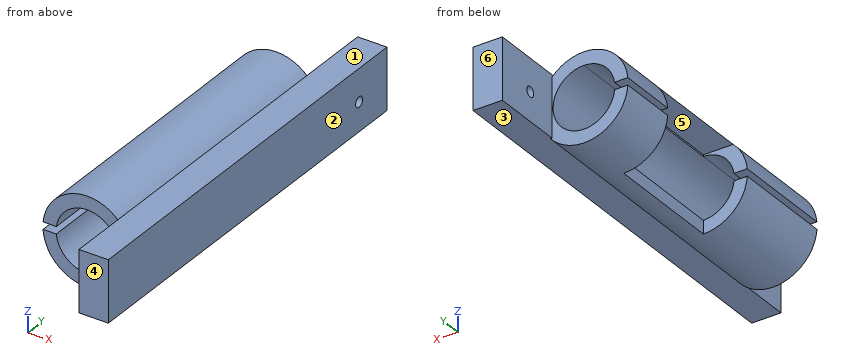
```python
from build123d import *

# Parameters (mm, degrees)
SKETCH_1_R           = 15
EXTRUDE_1_DEPTH      = 95
SKETCH_2_R           = 10.5
CUT_EXTRUDE_1_DEPTH  = 95
EXTRUDE_2_DEPTH      = 20
EXTRUDE_2_DEPTH_BACK = 120
SKETCH_3_W           = 10
SKETCH_3_H           = 20.861334049
SKETCH_7_W           = 15
SKETCH_7_H           = 40
CUT_EXTRUDE_3_DEPTH  = 125.54811794
SKETCH_8_W           = 8.046060948
SKETCH_8_H           = 2.469161561
CUT_EXTRUDE_4_DEPTH  = 118.826105551
SKETCH_10_R          = 1.75
CUT_EXTRUDE_5_DEPTH  = 124.649640842


with BuildPart() as part:
    # 草图1 → 凸台-拉伸1 (new body)
    with BuildSketch(Plane(origin=(0, 0, 0), x_dir=(1, 0, 0), z_dir=(0, 1, 0))):
        with Locations(Location((0, 0, 0), (0, 0, 270))):
            Circle(SKETCH_1_R)
    extrude(amount=EXTRUDE_1_DEPTH)

    # 草图2 → 切除-拉伸1 (cut)
    with BuildSketch(Plane(origin=(0, 95, 0), x_dir=(1, 0, 0), z_dir=(0, 1, 0))):
        with Locations(Location((0, 0, 0), (0, 0, 270))):
            Circle(SKETCH_2_R)
    extrude(amount=-CUT_EXTRUDE_1_DEPTH, mode=Mode.SUBTRACT)

    # 草图3 → 凸台-拉伸2 (add, two sides: drawn at the far end of the back side and taken through both)
    with BuildSketch(Plane(origin=(0, 0, 0), x_dir=(-1, 0, 0), z_dir=(0, -1, 0)).offset(-EXTRUDE_2_DEPTH_BACK)):
        with Locations((-15.808439379, -0.631614786)):
            Rectangle(SKETCH_3_W, SKETCH_3_H)
    extrude(amount=EXTRUDE_2_DEPTH + EXTRUDE_2_DEPTH_BACK)

    # 草图7 → 切除-拉伸3 (cut, through all)
    with BuildSketch(Plane.XY.offset(11.06228181)):
        with Locations((-7.5, 55)):
            Rectangle(SKETCH_7_W, SKETCH_7_H)
    extrude(amount=-CUT_EXTRUDE_3_DEPTH, mode=Mode.SUBTRACT)

    # 草图8 → 切除-拉伸4 (cut, through all)
    with BuildSketch(Plane(origin=(0, 95, 0), x_dir=(1, 0, 0), z_dir=(0, 1, 0))):
        with Locations((-13.909114393, -0.200189033)):
            Rectangle(SKETCH_8_W, SKETCH_8_H)
    extrude(amount=-CUT_EXTRUDE_4_DEPTH, mode=Mode.SUBTRACT)

    # 草图10 → 切除-拉伸5 (cut, through all)
    with BuildSketch(Plane.ZY.offset(-10.808439379)):
        with Locations((0, 106)):
            Circle(SKETCH_10_R)
    extrude(amount=-CUT_EXTRUDE_5_DEPTH, mode=Mode.SUBTRACT)


solid = part.part
```
CAD build for the part. Positions are in the model's coordinates, mm. Face numbers are marked on the shaded views. A direction names the side the tool comes from. Round coordinates to 2 decimals unless told otherwise and drop trailing zeros. Loops run counter-clockwise (first coordinate to the right, second up) from the corner with the lowest first, then second, coordinate; pieces in that order, holes last. Notation, with made-up numbers: (-24, 26.5) - (-20, 26.5) arc R25 ccw to (-20, 61.5) - close; hole circle Ø2 at (-19, 62). An arc over 180 degrees is marked (long way). Return JSON: item names as keys, results as strings. Group by question number.
Q1. Flat gauge pins, fed straight in: pin 1 Ø2 at (x, z) = (9, 12) entering from +Y; pin 2 Ø3 at (x, y) = (16, 20) entering from -Z; pin 3 Ø3.5 at (x, y) = (-12, 85) entering from +Z. Where does each tip first touch, or does it go through?
Q2. Band-saw the part on D-D on x = 15. Give the cut face in (y, z), plus the area to 3 significant figures.
Q3. Drill centre lines: line 1 along Z through (x, y) = (-0.5, 10); line 2 along X through (y, z) = (107.5, 5.75); line 3 along Z through (x, y) = (1.5, 22). Where is each one in solid material? Low to high. Write a range as [from, to].
Q4. Tool access for the marked faces 1 and 2: list every direction of +Z, -Z, +X, -X, +Y, -Y with a clear straight run to the whole face (end or side of a thin tool).
Q5. Band-saw the part on C-C on z = 5.25. Give the cut face in (x, y).
Q6. Band-saw the part on A-A on x = -12. Give the cut face in (y, z), plus the area to 3 significant figures.
Q7. Two-plate mould, pull along Y, no slides. Class the marked faces 3, 4, 5 and 6: +Y half, -Y half, draft (parallel to the pull), parting line (faces both ways), or undercut.
Q8. Band-saw the part on B-B on y = 106. Give the cut face in (x, z), plus the area to 3 significant figures.
Solutions:
{
 "1": {"pin 1": "stops at y = 95", "pin 2": "stops at z = -9.8", "pin 3": "stops at z = 10.95"},
 "2": {"outline": "(-20, -9.8) - (120, -9.8) - (120, 11.06) - (-20, 11.06) - close; hole circle Ø3.5 at (106, 0)", "area": "2,910 mm^2"},
 "3": {"line 1": "z = [-14.99, -10.49], [10.49, 14.99]", "line 2": "x = [10.81, 20.81]", "line 3": "z = [-14.92, -10.39], [10.39, 14.92]"},
 "4": {"face 1": "+Z, +X, +Y, -Y", "face 2": "+Z, -Z, +X, +Y, -Y"},
 "5": {"outline": "(-14.05, 0) - (-9.09, 0) - (-9.09, 35) - (-14.05, 35) - close; (-14.05, 75) - (-9.09, 75) - (-9.09, 95) - (-14.05, 95) - close; (9.09, 0) - (10.81, 0) - (10.81, -20) - (20.81, -20) - (20.81, 120) - (10.81, 120) - (10.81, 95) - (9.09, 95) - close"},
 "6": {"outline": "(0, -9) - (35, -9) - (35, -1.03) - (0, -1.03) - close; (0, 1.43) - (35, 1.43) - (35, 9) - (0, 9) - close; (75, -9) - (95, -9) - (95, -1.03) - (75, -1.03) - close; (75, 1.43) - (95, 1.43) - (95, 9) - (75, 9) - close", "area": "854 mm^2"},
 "7": {"face 3": "draft", "face 4": "-Y half", "face 5": "undercut", "face 6": "+Y half"},
 "8": {"outline": "(10.81, -9.8) - (20.81, -9.8) - (20.81, -1.75) - (10.81, -1.75) - close; (10.81, 1.75) - (20.81, 1.75) - (20.81, 11.06) - (10.81, 11.06) - close", "area": "174 mm^2"}
}
